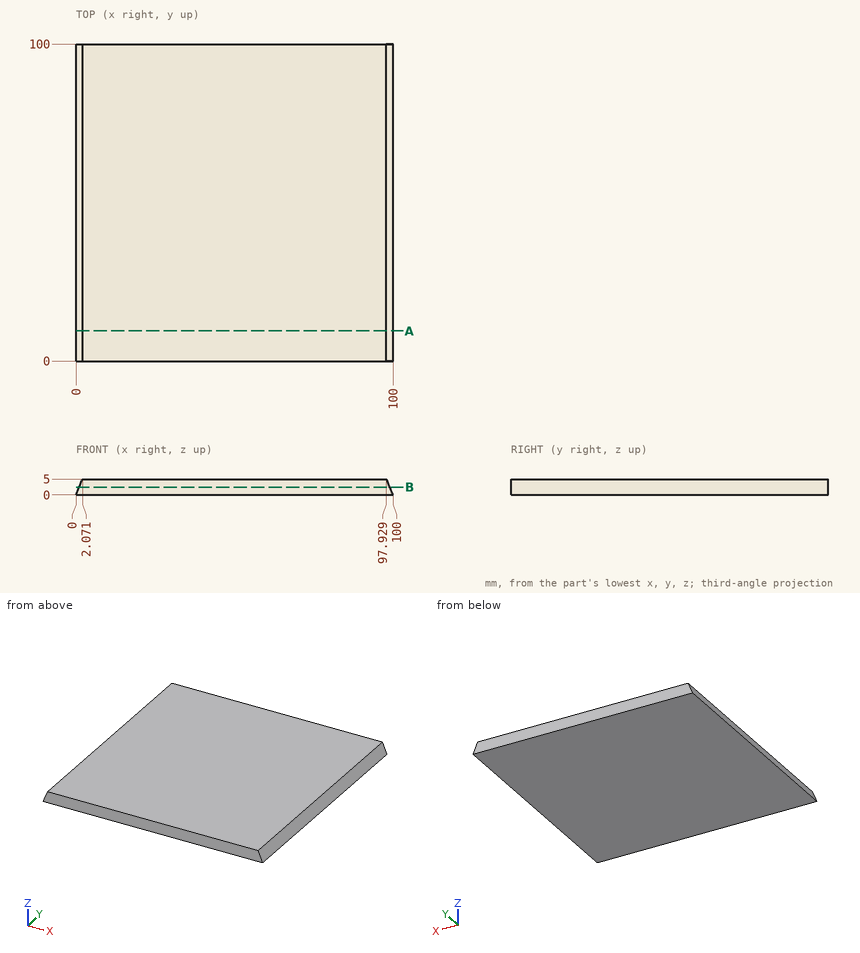
Geometry check sheet. Reference: drawing and pictorial views, mm from the part's lowest x, y, z. Coordinates: 2 decimals unless noted, no trailing zeros. Loops run counter-clockwise (first coordinate to the right, second up) from the corner with the lowest first, then second, coordinate; pieces in that order, holes last. Notation, with made-up numbers: (-37.75, 56) - (12.25, 56) arc R23 ccw to (12.25, 95) - close; hole circle Ø4 at (52.25, 46.25). An arc over 180 degrees is marked (long way). Return JSON: item names as keys, results as strings.
1. Go/stop test with a flat-tipped pin: pin 1 (1 mm diameter, centred on y = 19.5, z = 4.5, fed in from +X). Record where the tip stops, or that it passes through.
Established:
{"pin 1": "stops at x = 98.34"}
2. Section check A-A, the plane y = 9.5. Record the boundary of the cut face in (x, z), then the cut area to 3 significant figures.
Established:
{"outline": "(0, 0) - (100, 0) - (97.93, 5) - (2.07, 5) - close", "area": "490 mm2"}
3. Section check B-B, the plane z = 2.4. Record the boundary of the cut face in (x, y).
Established:
{"outline": "(0.99, 0) - (99.01, 0) - (99.01, 100) - (0.99, 100) - close"}
4. Thickness scan on L1, parallel to X at y = 75, z = 3.9; L2, parallel to X at y = 21.5, z = 2.35. Record the ranges inside material, lowest first.
Established:
{"L1": "x = 1.62 to 98.38", "L2": "x = 0.97 to 99.03"}
